Work out the finished part from the listing and answer in its coordinate system (mm). Face numbers are marked on the shaded views. A direction names the side the tool comes from. Coordinates: 2 decimals unless noted, no trailing zeros. Write each loop counter-clockwise with the first axis right and the second up, starting at its lowest first coordinate (ties: lowest second). Pieces come first, ordered by that corner, then holes. Notation, with made-up numbers: (14, -4.75) - (28, -4.75) arc R17 ccw to (28, 9.25) - close; hole circle Ø3 at (-3, 14.25). An arc over 180 degrees is marked (long way). Answer as a JSON object with one key per item and string values. Group by question number.
from build123d import *

# Parameters (mm, degrees)
F0_R     = 17.5
F0_W     = 23
F0_H     = 23
F1_DEPTH = 10
F2_R     = 1.5
F3_DEPTH = 25
F4_R     = 2.5
F5_DEPTH = 4


with BuildPart() as f1:
    # F0 (on Front) → F1 (new body)
    with BuildSketch(Plane.XZ):
        Circle(F0_R)
        Rectangle(F0_W, F0_H, mode=Mode.SUBTRACT)
    extrude(amount=F1_DEPTH)

    # F2 (on Top) → F3 (cut)
    with BuildSketch(Plane.XY):
        with Locations((0, -4)):
            Circle(F2_R)
    extrude(amount=-F3_DEPTH, mode=Mode.SUBTRACT)

    # F4 (on face) → F5 (cut)
    with BuildSketch(Plane.XY.offset(-11.5)):
        with Locations((0, -4)):
            Circle(F4_R)
    extrude(amount=-F5_DEPTH, mode=Mode.SUBTRACT)


solid = f1.part
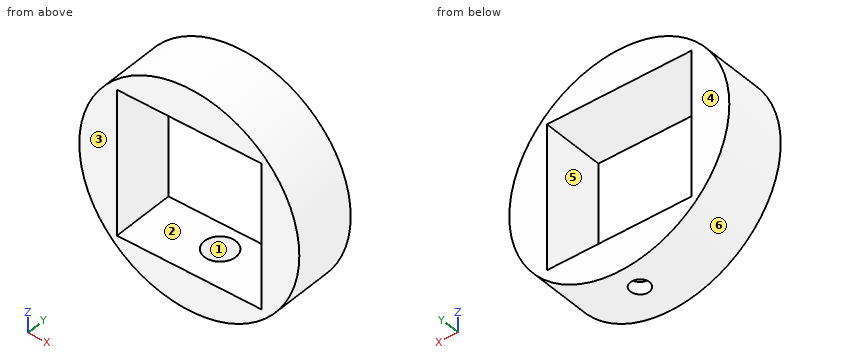
Q1. Section B-B on x = 0 is taken. Determine the outline of the cut face in (y, z), plus the area to 3 significant figures.
Q2. Section A-A on z = 0 is taken. Determine the outline of the cut face in (x, y), plus the area to 3 significant figures.
Q3. Consider L1, parallel to Z at x = -0.5, y = -0.75; L2, parallel to Y at x = 0, z = -13.35; L3, parallel to Y at x = 0, z = -16.1. Determine where each line is inside the solid, lowest interval first. Write a range as from..to.
Q4. Flat-ended cylindrical pins translate along their axes: pin 1 Ø4 at (x, y) = (3, -7) entering from +Z; pin 2 Ø2 at (x, y) = (11.5, -4) entering from -Z; pin 3 Ø4 at (y, z) = (-5.5, -4) entering from +X. Find the tip coordinate at first contact, or state that the pin passes through.
Q5. For a pull along Z with two mould halves and no side action, classify the marked faces 4, 5 and 6 as +Z half, -Z half, draft (parallel to the pull), parting line (faces both ways), or undercut.
Q6. A tool of negligible diameter and unlimited length cuts with its end or side. For the marked faces 1, 2 and 3, from which of +Z, -Z, +X, -X, +Y, -Y can it reach the whole face along a straight path? Write none if from no direction.
Q7. Section D-D on x = 7 is taken. Determine the outline of the cut face in (y, z), plus the area to 3 significant figures.
Q8. Section C-C on y = -9 is taken. Determine the outline of the cut face in (x, z).
Numbers:
{
 "1": {"outline": "(-10, -17.5) - (-5.5, -17.5) - (-5.5, -15.5) - (-6.5, -15.5) - (-6.5, -11.5) - (-10, -11.5) - close; (-10, 11.5) - (0, 11.5) - (0, 17.5) - (-10, 17.5) - close; (-2.5, -17.5) - (0, -17.5) - (0, -11.5) - (-1.5, -11.5) - (-1.5, -15.5) - (-2.5, -15.5) - close", "area": "94.0 mm²"},
 "2": {"outline": "(-17.5, -10) - (-11.5, -10) - (-11.5, 0) - (-17.5, 0) - close; (11.5, -10) - (17.5, -10) - (17.5, 0) - (11.5, 0) - close", "area": "120 mm²"},
 "3": {"L1": "z = -17.49..-11.5, 11.5..17.49", "L2": "y = -10..-6.5, -1.5..0", "L3": "y = -10..-5.5, -2.5..0"},
 "4": {"pin 1": "stops at z = 17.47", "pin 2": "stops at z = -14", "pin 3": "stops at x = 17.39"},
 "5": {"face 4": "draft", "face 5": "undercut", "face 6": "parting line"},
 "6": {"face 1": "none", "face 2": "+Y, -Y", "face 3": "+Z, -Z, +X, -X, -Y"},
 "7": {"outline": "(-10, -16.04) - (0, -16.04) - (0, -11.5) - (-10, -11.5) - close; (-10, 11.5) - (0, 11.5) - (0, 16.04) - (-10, 16.04) - close", "area": "90.8 mm²"},
 "8": {"outline": "circle Ø35 at (0, 0); hole (-11.5, -11.5) - (11.5, -11.5) - (11.5, 11.5) - (-11.5, 11.5) - close"}
}
